Source: CAD feature listing. Evaluate the final solid. Frame: model axes, mm. A direction names the side the tool comes from. Round coordinates to 2 decimals unless told otherwise and drop trailing zeros. Loops run counter-clockwise (first coordinate to the right, second up) from the corner with the lowest first, then second, coordinate; pieces in that order, holes last. Notation, with made-up numbers: M 45.5,3.5 L 67.5,3.5 A28 cw 67.5,29.5 Z; hole C 11.5,-3 d7. An arc over 180 degrees is marked long. Write each question's results on one line, items separated by ' | '. Start each with the question number.
1. Section B-B on x = 0. Output: boundary loops of the cut face in (y, z), and give its area (3 significant figures).
2. Set-up query: faces 4 (the flat face through (-8, 0, 5)), 5 (the flat face through (10.85, 6.52, 16.09)). Return all of +Z, -Z, +X, -X, +Y, -Y with unobstructed straight access to the full face (end or side cutting, diameter ignored); none if empty.
3. Contact query for a flat-ended pin moving along its axis: pin 1 Ø16.5 at (x, z) = (0, 0) entering from +Y. Output: stop coordinate, or through.
4. Ray query, line 1 (X direction, y = 0.55, z = 0); line 2 (X direction, y = 2.5, z = 0); line 3 (Z direction, x = 9, y = 7). Return the intervals inside material, ascending.
5. Section C-C on y = 3. Output: boundary loops of the cut face in (x, z), and give its area (3 significant figures).
6. Draft query along Z for faces 1 (the flat face through (0, 4, -21)), 2 (the flat face through (-32.5, 4, 0)), 3 (the cylindrical face through (-9.71, 3.65, -16.75)). Return one class per face: released by +Z, released by -Z, zero draft, split by the parting line, or undercut.
7. Section A-A on y = 6. Output: boundary loops of the cut face in (x, z).
from build123d import *

# Parameters (mm, degrees)
SCHIZZO1_R                        = 27
ESTRUSIONE_ESTRUSIONE1_DEPTH      = 1
SCHIZZO2_R                        = 8
TAGLIO_ESTRUSIONE1_DEPTH          = 39.19685851
SCHIZZO3_R                        = 27
SCHIZZO3_R_2                      = 13.6
ESTRUSIONE_ESTRUSIONE2_DEPTH      = 5
ESTRUSIONE_ESTRUSIONE3_DEPTH      = 2
ESTRUSIONE_ESTRUSIONE3_DEPTH_BACK = 1
SCHIZZO5_W                        = 65
SCHIZZO5_H                        = 42
SCHIZZO5_R                        = 13.6
TAGLIO_ESTRUSIONE2_START          = -27
TAGLIO_ESTRUSIONE2_OUTLINE_R      = 1.35
TAGLIO_ESTRUSIONE2_DEPTH          = 53.999999754
TAGLIO_ESTRUSIONE3_DEPTH          = 44.869308585
TAGLIO_ESTRUSIONE3_DEPTH_BACK     = 44.869308585
SCHIZZO8_W                        = 81.46070362
SCHIZZO8_H                        = 59.010327036
SCHIZZO8_W_2                      = 65
SCHIZZO8_H_2                      = 42
TAGLIO_ESTRUSIONE5_DEPTH          = 43.676105804
SCHIZZO10_W                       = 15.529437252
SCHIZZO10_H                       = 42
ESTRUSIONE_ESTRUSIONE4_DEPTH      = 5
SCHIZZO11_W                       = 15.529437252
SCHIZZO11_H                       = 42
ESTRUSIONE_ESTRUSIONE5_DEPTH      = 5


# Read off the part's stored shape, not the designer's step: Taglio-Estrusione2
with BuildPart() as part:
    # Schizzo1 → Estrusione-Estrusione1 (new body)
    with BuildSketch(Plane(origin=(0, 0, 0), x_dir=(1, 0, 0), z_dir=(0, 1, 0))):
        with Locations(Location((0, 0, 0), (0, 0, 270))):
            Circle(SCHIZZO1_R)
    extrude(amount=ESTRUSIONE_ESTRUSIONE1_DEPTH)

    # Schizzo2 → Taglio-Estrusione1 (cut, through all)
    with BuildSketch(Plane(origin=(0, 1, 0), x_dir=(1, 0, 0), z_dir=(0, 1, 0))):
        with Locations(Location((0, 0, 0), (0, 0, 270))):
            Circle(SCHIZZO2_R)
    extrude(amount=-TAGLIO_ESTRUSIONE1_DEPTH, mode=Mode.SUBTRACT)

    # Schizzo3 → Estrusione-Estrusione2 (add)
    with BuildSketch(Plane(origin=(0, 1, 0), x_dir=(1, 0, 0), z_dir=(0, 1, 0))):
        with Locations(Location((0, 0, 0), (0, 0, 270))):
            Circle(SCHIZZO3_R)
        with Locations(Location((0, 0, 0), (0, 0, 270))):
            Circle(SCHIZZO3_R_2, mode=Mode.SUBTRACT)
    extrude(amount=ESTRUSIONE_ESTRUSIONE2_DEPTH)

    # Schizzo5 → Estrusione-Estrusione3 (add, two sides: drawn at the far end of the back side and taken through both)
    with BuildSketch(Plane(origin=(0, 6, 0), x_dir=(1, 0, 0), z_dir=(0, 1, 0)).offset(-ESTRUSIONE_ESTRUSIONE3_DEPTH_BACK)):
        Rectangle(SCHIZZO5_W, SCHIZZO5_H)
        with Locations(Location((0, 0, 0), (0, 0, 270))):
            Circle(SCHIZZO5_R, mode=Mode.SUBTRACT)
    extrude(amount=ESTRUSIONE_ESTRUSIONE3_DEPTH + ESTRUSIONE_ESTRUSIONE3_DEPTH_BACK)

    # Taglio-Estrusione2 outline → Taglio-Estrusione2 (cut)
    with BuildSketch(Plane(origin=(0, 0, 0), x_dir=(0.866025403784438, 0, -0.500000000000001), z_dir=(0.500000000000001, 0, 0.866025403784438)).offset(TAGLIO_ESTRUSIONE2_START)):
        with Locations((0, 5)):
            Circle(TAGLIO_ESTRUSIONE2_OUTLINE_R)
    extrude(amount=TAGLIO_ESTRUSIONE2_DEPTH, mode=Mode.SUBTRACT)

    # Schizzo3D2 → Taglio-Estrusione3 (cut, two sides: drawn at the far end of the back side and taken through both)
    with BuildSketch(Plane(origin=(1.169134295, 5, -0.675), x_dir=(-0.41149103074101084, 0.8799053976571924, 0.23757445736745078), z_dir=(-0.5000000000000011, 1.0747888534457561e-14, -0.866025403784438)).offset(-TAGLIO_ESTRUSIONE3_DEPTH_BACK)):
        Polygon((0, 0), (1.28290207, -2.375744574), (5.682429058, 0), (4.399526988, 2.375744574), align=None)
    extrude(amount=TAGLIO_ESTRUSIONE3_DEPTH + TAGLIO_ESTRUSIONE3_DEPTH_BACK, mode=Mode.SUBTRACT)

    # Schizzo8 → Taglio-Estrusione5 (cut, through all)
    with BuildSketch(Plane(origin=(0, 6, 0), x_dir=(1, 0, 0), z_dir=(0, 1, 0))):
        Rectangle(SCHIZZO8_W, SCHIZZO8_H)
        Rectangle(SCHIZZO8_W_2, SCHIZZO8_H_2, mode=Mode.SUBTRACT)
    extrude(amount=-TAGLIO_ESTRUSIONE5_DEPTH, mode=Mode.SUBTRACT)

    # Schizzo10 → Estrusione-Estrusione4 (add)
    with BuildSketch(Plane.XZ.offset(-5)):
        with Locations((-24.735281374, 0)):
            Rectangle(SCHIZZO10_W, SCHIZZO10_H)
    extrude(amount=ESTRUSIONE_ESTRUSIONE4_DEPTH)

    # Schizzo11 → Estrusione-Estrusione5 (add)
    with BuildSketch(Plane.XZ.offset(-5)):
        with Locations((24.735281374, 0)):
            Rectangle(SCHIZZO11_W, SCHIZZO11_H)
    extrude(amount=ESTRUSIONE_ESTRUSIONE5_DEPTH)


solid = part.part
Taken from the geometry:
1) outline: M 0,-21 L 8,-21 L 8,-13.6 L 1,-13.6 L 1,-8 L 0,-8 Z; M 0,8 L 1,8 L 1,13.6 L 8,13.6 L 8,21 L 0,21 Z | area: 130 mm^2
2) face 4: +Z, -Z, +X, -X, -Y | face 5: +Y
3) pin 1: y = 1
4) line 1: -32.5 to -8, 8 to 32.5 | line 2: -32.5 to -13.6, 13.6 to 32.5 | line 3: -21 to -10.2, 10.2 to 12.89, 18.29 to 21
5) outline: M -32.5,-21 L 32.5,-21 L 32.5,21 L -32.5,21 Z; hole C 0,0 d27.2 | area: 2,150 mm^2
6) face 1: released by -Z | face 2: zero draft | face 3: undercut
7) outline: M -32.5,-21 L -13.68,-21 L -7.94,-11.04 A13.6 cw 5.6,12.39 L 10.57,21 L -32.5,21 Z; M -10.57,-21 L 32.5,-21 L 32.5,21 L 13.68,21 L 7.94,11.04 A13.6 cw -5.6,-12.39 Z
